```python
from build123d import *
from build123d.topology import SkipClean

# Parameters (mm, degrees)
SKETCH2_R            = 11.25
SKETCH2_R_2          = 1.55
SKETCH2_R_3          = 2.1
BOSS_EXTRUDE1_DEPTH  = 4
SKETCH3_W            = 57.5
SKETCH3_H            = 14
SKETCH3_W_2          = 43
SKETCH3_H_2          = 43
BOSS_EXTRUDE2_DEPTH  = 10
SKETCH4_W            = 63.5
SKETCH4_H            = 20
SKETCH4_R            = 2.1
BOSS_EXTRUDE3_DEPTH  = 4
BOSS_EXTRUDE4_DEPTH  = 10
SKETCH6_W            = 20
SKETCH6_H            = 40
CUT_EXTRUDE1_DEPTH   = 31
SKETCH7_W            = 3
SKETCH7_H            = 40
BOSS_EXTRUDE5_DEPTH  = 10
SKETCH8_W            = 20
SKETCH8_H            = 40
CUT_EXTRUDE2_DEPTH   = 31
SKETCH9_W            = 3
SKETCH9_H            = 34
BOSS_EXTRUDE6_DEPTH  = 10
SKETCH10_R           = 2.1
CUT_EXTRUDE3_DEPTH   = 31
BOSS_EXTRUDE7_DEPTH  = 4
SKETCH12_W           = 0.5
SKETCH12_H           = 14
CUT_EXTRUDE4_DEPTH   = 31
SKETCH13_W           = 3
SKETCH13_H           = 34
BOSS_EXTRUDE8_DEPTH  = 10
SKETCH15_R           = 2.1
BOSS_EXTRUDE9_DEPTH  = 4
SKETCH16_W           = 14
SKETCH16_H           = 34
SKETCH16_H_2         = 3
BOSS_EXTRUDE10_DEPTH = 10
SKETCH17_W           = 53
SKETCH17_H           = 3.5
BOSS_EXTRUDE11_DEPTH = 14
SKETCH19_W           = 43
SKETCH19_H           = 43
SKETCH19_W_2         = 14
SKETCH19_H_2         = 14
BOSS_EXTRUDE12_DEPTH = 6
SKETCH20_W           = 14
SKETCH20_H           = 14
CUT_EXTRUDE5_DEPTH   = 6
SKETCH21_W           = 14
SKETCH21_H           = 14
SKETCH21_R           = 2.1
SKETCH21_R_2         = 2.6
BOSS_EXTRUDE13_DEPTH = 4


with BuildPart() as part:
    # Sketch2 → Boss-Extrude1 (new body)
    with BuildSketch(Plane(origin=(0, 0, 0), x_dir=(1, 0, 0), z_dir=(0, 1, 0))):
        Polygon((-26.5, 26.5), (26.5, 26.5), (26.5, 10), (90, 10), (90, -10), (26.5, -10), (26.5, -26.5), (-26.5, -26.5), align=None)
        with Locations(Location((0, 0, 0), (0, 0, 270))):
            Circle(SKETCH2_R, mode=Mode.SUBTRACT)
        with Locations(Location((-15.5, 15.5, 0), (0, 0, 270))):
            Circle(SKETCH2_R_2, mode=Mode.SUBTRACT)
        with Locations(Location((15.5, 15.5, 0), (0, 0, 270))):
            Circle(SKETCH2_R_2, mode=Mode.SUBTRACT)
        with Locations(Location((15.5, -15.5, 0), (0, 0, 270))):
            Circle(SKETCH2_R_2, mode=Mode.SUBTRACT)
        with Locations(Location((-15.5, -15.5, 0), (0, 0, 270))):
            Circle(SKETCH2_R_2, mode=Mode.SUBTRACT)
        with Locations(Location((40, 0, 0), (0, 0, 270))):
            Circle(SKETCH2_R_3, mode=Mode.SUBTRACT)
        with Locations(Location((60, 0, 0), (0, 0, 270))):
            Circle(SKETCH2_R_3, mode=Mode.SUBTRACT)
        with Locations(Location((80, 0, 0), (0, 0, 270))):
            Circle(SKETCH2_R_3, mode=Mode.SUBTRACT)
    extrude(amount=BOSS_EXTRUDE1_DEPTH)

    # Sketch3 → Boss-Extrude2 (add)
    with BuildSketch(Plane(origin=(0, 0, 0), x_dir=(1, 0, 0), z_dir=(0, 1, 0))):
        Polygon((-26.5, -26.5), (26.5, -26.5), (26.5, -10), (90, -10), (90, 10), (26.5, 10), (26.5, 26.5), (-26.5, 26.5), align=None)
        with Locations((58.25, 0)):
            Rectangle(SKETCH3_W, SKETCH3_H, mode=Mode.SUBTRACT)
        Rectangle(SKETCH3_W_2, SKETCH3_H_2, mode=Mode.SUBTRACT)
    extrude(amount=-BOSS_EXTRUDE2_DEPTH)

    # Sketch4 → Boss-Extrude3 (add)
    with BuildSketch(Plane(origin=(0, 4, 0), x_dir=(1, 0, 0), z_dir=(0, 1, 0))):
        with Locations((58.25, 20)):
            Rectangle(SKETCH4_W, SKETCH4_H)
        with Locations(Location((80, 20, 0), (0, 0, 270))):
            Circle(SKETCH4_R, mode=Mode.SUBTRACT)
        with Locations(Location((60, 20, 0), (0, 0, 270))):
            Circle(SKETCH4_R, mode=Mode.SUBTRACT)
        with Locations(Location((40, 20, 0), (0, 0, 270))):
            Circle(SKETCH4_R, mode=Mode.SUBTRACT)
    extrude(amount=-BOSS_EXTRUDE3_DEPTH)

    # Sketch5 → Boss-Extrude4 (add)
    with BuildSketch(Plane.XZ):
        Polygon((90, -10), (26.5, -10), (26.5, -26.5), (26.5, -30), (90, -30), align=None)
        Polygon((87, -13), (29.5, -13), (29.5, -26.5), (29.5, -27), (87, -27), align=None, mode=Mode.SUBTRACT)
    extrude(amount=BOSS_EXTRUDE4_DEPTH)

    # Sketch6 → Cut-Extrude1 (cut)
    with BuildSketch(Plane.XZ.offset(10)):
        with Locations((80, -10)):
            Rectangle(SKETCH6_W, SKETCH6_H)
    extrude(amount=-CUT_EXTRUDE1_DEPTH, mode=Mode.SUBTRACT)

    # Sketch7 → Boss-Extrude5 (add)
    with BuildSketch(Plane.XZ):
        with Locations((68.5, -10)):
            Rectangle(SKETCH7_W, SKETCH7_H)
    extrude(amount=BOSS_EXTRUDE5_DEPTH)

    # Sketch8 → Cut-Extrude2 (cut)
    with BuildSketch(Plane.XZ.offset(10)):
        with Locations((60, -10)):
            Rectangle(SKETCH8_W, SKETCH8_H)
    extrude(amount=-CUT_EXTRUDE2_DEPTH, mode=Mode.SUBTRACT)

    # Sketch9 → Boss-Extrude6 (add)
    with BuildSketch(Plane.XZ):
        with Locations((48.5, -10)):
            Rectangle(SKETCH9_W, SKETCH9_H)
    extrude(amount=BOSS_EXTRUDE6_DEPTH)

    # Sketch10 → Cut-Extrude3 (cut)
    with BuildSketch(Plane.XZ.offset(10)):
        with Locations((36.5, -20)):
            Circle(SKETCH10_R)
        with Locations((36.5, 0)):
            Circle(SKETCH10_R)
    extrude(amount=-CUT_EXTRUDE3_DEPTH, mode=Mode.SUBTRACT)

    # Sketch11 → Boss-Extrude7 (add)
    with SkipClean():  # the faces are left unmerged after this step: merging them gives an invalid solid
        with BuildSketch(Plane.XZ):
            with BuildLine():
                ThreePointArc((38.25, -18.839181323), (38.6, -20), (38.25, -21.160818677))
                ThreePointArc((38.25, -21.160818677), (42.1, -20), (38.25, -18.839181323))
            make_face()
            with BuildLine():
                ThreePointArc((38.25, -1.160818677), (42.1, 0), (38.25, 1.160818677))
                ThreePointArc((38.25, 1.160818677), (38.6, 0), (38.25, -1.160818677))
            make_face()
        extrude(amount=-BOSS_EXTRUDE7_DEPTH)

    # Sketch12 → Cut-Extrude4 (cut)
    with SkipClean():  # the faces are left unmerged after this step: merging them gives an invalid solid
        with BuildSketch(Plane.XZ.offset(10)):
            Polygon((50, -30), (46.5, -30), (46.5, -36.524115579), (58.005951577, -36.524115579), (58.005951577, 17.068151821), (46.5, 17.068151821), (46.5, 10), (50, 10), align=None)
            Polygon((47, -27), (46.5, -27), (46.5, -30), (50, -30), (50, 10), (46.5, 10), (46.5, 7), (47, 7), (47, -7), (46.5, -7), (46.5, -13), (47, -13), align=None)
            Polygon((46.5, -13), (46.5, -20), (46.5, -27), (47, -27), (47, -13), align=None)
            with Locations((46.75, 0)):
                Rectangle(SKETCH12_W, SKETCH12_H)
        extrude(amount=-CUT_EXTRUDE4_DEPTH, mode=Mode.SUBTRACT)

    # Sketch13 → Boss-Extrude8 (add)
    with SkipClean():  # the faces are left unmerged after this step: merging them gives an invalid solid
        with BuildSketch(Plane.XZ):
            with Locations((45, -10)):
                Rectangle(SKETCH13_W, SKETCH13_H)
        extrude(amount=BOSS_EXTRUDE8_DEPTH)

    # Sketch15 → Boss-Extrude9 (add)
    with SkipClean():  # the faces are left unmerged after this step: merging them gives an invalid solid
        with BuildSketch(Plane(origin=(0, 4, 0), x_dir=(1, 0, 0), z_dir=(0, 1, 0))):
            Polygon((-26.5, 30), (-46.5, 30), (-46.5, -10), (-26.5, -10), (-26.5, 26.5), align=None)
            with Locations(Location((-36.5, 0, 0), (0, 0, 270))):
                Circle(SKETCH15_R, mode=Mode.SUBTRACT)
            with Locations(Location((-36.5, 20, 0), (0, 0, 270))):
                Circle(SKETCH15_R, mode=Mode.SUBTRACT)
        extrude(amount=-BOSS_EXTRUDE9_DEPTH)

    # Sketch16 → Boss-Extrude10 (add)
    # profile 1 of 3: a face of its own
    with SkipClean():  # the faces are left unmerged after this step: merging them gives an invalid solid
        with BuildSketch(Plane.XZ):
            Polygon((-46.5, 10), (-46.5, -30), (-26.5, -30), (-26.5, -26.5), (-26.5, 10), align=None)
            with Locations((-36.5, -10)):
                Rectangle(SKETCH16_W, SKETCH16_H, mode=Mode.SUBTRACT)
        # profile 2 of 3: a face of its own
        with BuildSketch(Plane.XZ):
            with Locations((-36.5, -11.5)):
                Rectangle(SKETCH16_W, SKETCH16_H_2)
        # profile 3 of 3: a face of its own
        with BuildSketch(Plane.XZ):
            with Locations((-36.5, -8.5)):
                Rectangle(SKETCH16_W, SKETCH16_H_2)
        extrude(amount=BOSS_EXTRUDE10_DEPTH)

    # Sketch17 → Boss-Extrude11 (add)
    with SkipClean():  # the faces are left unmerged after this step: merging them gives an invalid solid
        with BuildSketch(Plane.XZ.offset(10)):
            with Locations((0, -28.25)):
                Rectangle(SKETCH17_W, SKETCH17_H)
        extrude(amount=-BOSS_EXTRUDE11_DEPTH)

    # Sketch19 → Boss-Extrude12 (add)
    with SkipClean():  # the faces are left unmerged after this step: merging them gives an invalid solid
        with BuildSketch(Plane.XZ.offset(10)):
            Polygon((-46.5, 10), (-46.5, -30), (46.5, -30), (46.5, 10), (26.5, 10), (26.5, 26.5), (-26.5, 26.5), (-26.5, 10), align=None)
            Rectangle(SKETCH19_W, SKETCH19_H, mode=Mode.SUBTRACT)
            with Locations((36.5, -20)):
                Rectangle(SKETCH19_W_2, SKETCH19_H_2, mode=Mode.SUBTRACT)
            with Locations((36.5, 0)):
                Rectangle(SKETCH19_W_2, SKETCH19_H_2, mode=Mode.SUBTRACT)
            with Locations((-36.5, -20)):
                Rectangle(SKETCH19_W_2, SKETCH19_H_2, mode=Mode.SUBTRACT)
            with Locations((-36.5, 0)):
                Rectangle(SKETCH19_W_2, SKETCH19_H_2, mode=Mode.SUBTRACT)
        extrude(amount=BOSS_EXTRUDE12_DEPTH)

    # Sketch20 → Cut-Extrude5 (cut)
    with SkipClean():  # the faces are left unmerged after this step: merging them gives an invalid solid
        with BuildSketch(Plane.XZ):
            with Locations((-36.5, -20)):
                Rectangle(SKETCH20_W, SKETCH20_H)
            with Locations((-36.5, 0)):
                Rectangle(SKETCH20_W, SKETCH20_H)
        extrude(amount=-CUT_EXTRUDE5_DEPTH, mode=Mode.SUBTRACT)

    # Sketch21 → Boss-Extrude13 (add)
    # profile 1 of 2: a face of its own
    with SkipClean():  # the faces are left unmerged after this step: merging them gives an invalid solid
        with BuildSketch(Plane.XZ.offset(16)):
            with Locations((-36.5, -20)):
                Rectangle(SKETCH21_W, SKETCH21_H)
            with Locations(Location((-36.5, -20, 0), (0, 0, 270))):
                Circle(SKETCH21_R, mode=Mode.SUBTRACT)
        # profile 2 of 2: a face of its own
        with BuildSketch(Plane.XZ.offset(16)):
            with Locations((-36.5, 0)):
                Rectangle(SKETCH21_W, SKETCH21_H)
            with Locations(Location((-36.5, 0, 0), (0, 0, 270))):
                Circle(SKETCH21_R_2, mode=Mode.SUBTRACT)
        extrude(amount=-BOSS_EXTRUDE13_DEPTH)


solid = part.part
```
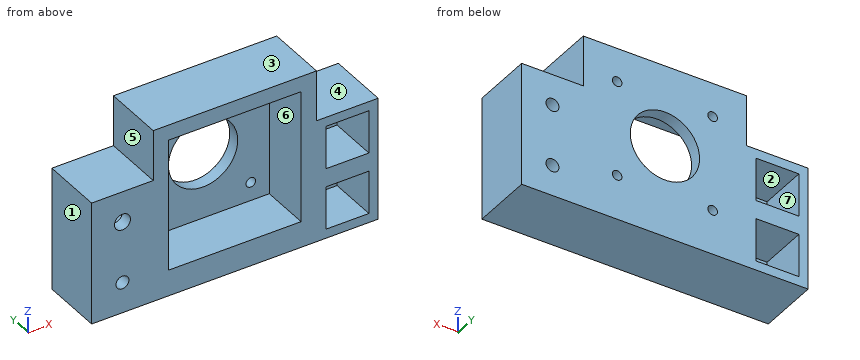
The listing builds one solid part. Answer for the finished solid, in the listing's coordinates (mm). Face numbers are marked on the shaded views. A direction names the side the tool comes from. Coordinates: 2 decimals unless noted, no trailing zeros. Write each loop counter-clockwise with the first axis right and the second up, starting at its lowest first coordinate (ties: lowest second). Pieces come first, ordered by that corner, then holes. Notation, with made-up numbers: (82.25, 16.25) - (108.25, 16.25) arc R21 ccw to (108.25, 32.25) - close; hole circle Ø5 at (-38, -32). An arc over 180 degrees is marked (long way). Return JSON: item names as keys, results as strings. Group by question number.
1. A cutting plane is placed at B-B, the plane z = -15.5. Determine the outline of the cut face in (x, y), plus the area to 3 significant figures.
2. Which of the six approach directions +Z, -Z, +X, -X, +Y, -Y give full straight-line access (tool end or side, diameter ignored) to the marked faces 4, 5, 6 and 7?
3. A cutting plane is placed at D-D, the plane x = 36.5. Determine the outline of the cut face in (y, z).
4. Given pin 1 (5 mm diameter, centred on y = -2, z = 16.5, fed in from -X); pin 2 (6 mm diameter, centred on x = -36.5, z = 0, fed in from +Y); pin 3 (4 mm diameter, centred on x = -35.5, y = -1, fed in from +Z); pin 4 (11 mm diameter, centred on x = -39.5, z = -22, fed in from +Y), each flat-ended and moving along its own axis, determine where each tip first touches the part or whether it passes through.
5. A cutting plane is placed at A-A, the plane x = -15.5. Determine the outline of the cut face in (y, z), plus the area to 3 significant figures.
6. Straight lines are drawn through the part: L1, parallel to X at y = 1.5, z = -15.5; L2, parallel to X at y = 3, z = 15.5; L3, parallel to X at y = -3, z = -20. For each, find the intervals that lie inside material, in ascending order.
7. A cutting plane is placed at C-C, the plane y = -13.25. Determine the outline of the cut face in (x, z).
8. Determine the mould class of the marked faces 1, 2 and 3 for opening direction X: released by +X, released by -X, zero draft, split by the parting line, or undercut.
Ans:
{
 "1": {"outline": "(-46.5, -16) - (-21.5, -16) - (-21.5, 0) - (-17.05, 0) - (-17.05, 4) - (-29.5, 4) - (-29.5, -12) - (-43.5, -12) - (-43.5, 4) - (-46.5, 4) - close; (-13.95, 0) - (13.95, 0) - (13.95, 4) - (-13.95, 4) - close; (17.05, 0) - (21.5, 0) - (21.5, -16) - (29.5, -16) - (29.5, 0) - (43.5, 0) - (43.5, -16) - (46.5, -16) - (46.5, 4) - (17.05, 4) - close", "area": "699 mm²"},
 "2": {"face 4": "+Z, +X, +Y, -Y", "face 5": "+Z, -X, +Y, -Y", "face 6": "-Y", "face 7": "+Y"},
 "3": {"outline": "(-16, -30) - (4, -30) - (4, -22.1) - (0, -22.1) - (0, -27) - (-16, -27) - close; (-16, -13) - (0, -13) - (0, -17.9) - (4, -17.9) - (4, -2.1) - (0, -2.1) - (0, -7) - (-16, -7) - close; (-16, 7) - (0, 7) - (0, 2.1) - (4, 2.1) - (4, 10) - (-16, 10) - close"},
 "4": {"pin 1": "x = -26.5", "pin 2": "y = -12", "pin 3": "z = 10", "pin 4": "y = 4"},
 "5": {"outline": "(-16, -30) - (4, -30) - (4, -17.05) - (0, -17.05) - (0, -21.5) - (-16, -21.5) - close; (-16, 21.5) - (0, 21.5) - (0, 17.05) - (4, 17.05) - (4, 26.5) - (-16, 26.5) - close; (0, -13.95) - (4, -13.95) - (4, 13.95) - (0, 13.95) - close", "area": "417 mm²"},
 "6": {"L1": "-46.5 to -43.5, -29.5 to -17.05, -13.95 to 13.95, 17.05 to 46.5", "L2": "-26.5 to -17.05, -13.95 to 13.95, 17.05 to 26.5", "L3": "-46.5 to -43.5, -29.5 to -21.5, 21.5 to 29.5, 43.5 to 46.5"},
 "7": {"outline": "(-46.5, -30) - (46.5, -30) - (46.5, 10) - (26.5, 10) - (26.5, 26.5) - (-26.5, 26.5) - (-26.5, 10) - (-46.5, 10) - close; hole circle Ø5.2 at (-36.5, 0); hole circle Ø4.2 at (-36.5, -20); hole (-21.5, -21.5) - (21.5, -21.5) - (21.5, 21.5) - (-21.5, 21.5) - close; hole (29.5, -27) - (43.5, -27) - (43.5, -13) - (29.5, -13) - close; hole (29.5, -7) - (43.5, -7) - (43.5, 7) - (29.5, 7) - close"},
 "8": {"face 1": "released by -X", "face 2": "undercut", "face 3": "zero draft"}
}
